For this review, take the finished solid that the model builds, in its own axes (mm). A direction names the side the tool comes from. Give positions to 0.01 mm unless a question says otherwise; leave off trailing zeros. Loops run counter-clockwise (first coordinate to the right, second up) from the corner with the lowest first, then second, coordinate; pieces in that order, holes last.
```python
from build123d import *

# Parameters (mm, degrees)
F0_R     = 3.5
F0_R_2   = 1.5
F1_DEPTH = 2
F0_W     = 22.5
F0_H     = 32
F2_DEPTH = 4
F3_DEPTH = 1


with BuildPart() as f1:
    # F0 (on Top) → F1 (new body)
    with BuildSketch(Plane.XY):
        with BuildLine():
            ThreePointArc((20, 26.114874), (18.904278, 28.704066), (16.409269, 30))
            Line((16.409269, 30), (-16.409269, 30))
            ThreePointArc((-16.409269, 30), (-18.904278, 28.704066), (-20, 26.114874))
            Line((-20, 26.114874), (-20, 24.938533))
            ThreePointArc((-20, 24.938533), (-19.396294, 22.556811), (-17.73096, 20.750233))
            Line((-17.73096, 20.750233), (-13, 17.665434))
            Line((-13, 17.665434), (-13, 18))
            Line((-13, 18), (13, 18))
            Line((13, 18), (13, 17.665434))
            Line((13, 17.665434), (17.73096, 20.750233))
            ThreePointArc((17.73096, 20.750233), (19.396294, 22.556811), (20, 24.938533))
            Line((20, 24.938533), (20, 26.114874))
        make_face()
        with Locations((-15, 25)):
            Circle(F0_R, mode=Mode.SUBTRACT)
        Polygon((-9.18, 27), (-9.18, 28), (-8.18, 28), (8.18, 28), (9.170838, 28), (9.170838, 27), (9.170838, 21), (9.170838, 20), (8.18, 20), (-8.18, 20), (-9.18, 20), (-9.18, 21), align=None, mode=Mode.SUBTRACT)
        with Locations((15, 25)):
            Circle(F0_R, mode=Mode.SUBTRACT)
        with BuildLine():
            Line((17.73096, -20.750233), (13, -17.665434))
            Line((13, -17.665434), (13, -18))
            Line((13, -18), (-13, -18))
            Line((-13, -18), (-13, -17.665434))
            Line((-13, -17.665434), (-17.73096, -20.750233))
            ThreePointArc((-17.73096, -20.750233), (-19.396294, -22.556811), (-20, -24.938533))
            Line((-20, -24.938533), (-20, -26.114874))
            ThreePointArc((-20, -26.114874), (-18.904278, -28.704066), (-16.409269, -30))
            Line((-16.409269, -30), (16.409269, -30))
            ThreePointArc((16.409269, -30), (18.904278, -28.704066), (20, -26.114874))
            Line((20, -26.114874), (20, -24.938533))
            ThreePointArc((20, -24.938533), (19.396294, -22.556811), (17.73096, -20.750233))
        make_face()
        with Locations((-15, -25)):
            Circle(F0_R, mode=Mode.SUBTRACT)
        Polygon((-8.18, -20), (8.18, -20), (9.170838, -20), (9.170838, -21), (9.170838, -27), (9.170838, -28), (8.18, -28), (-8.18, -28), (-9.18, -28), (-9.18, -27), (-9.18, -21), (-9.18, -20), align=None, mode=Mode.SUBTRACT)
        with Locations((15, -25)):
            Circle(F0_R, mode=Mode.SUBTRACT)
        with Locations((-15, -25)):
            Circle(F0_R)
        with Locations((-15, -25)):
            Circle(F0_R_2, mode=Mode.SUBTRACT)
        with Locations((15, -25)):
            Circle(F0_R)
        with Locations((15, -25)):
            Circle(F0_R_2, mode=Mode.SUBTRACT)
        with Locations((15, 25)):
            Circle(F0_R)
        with Locations((15, 25)):
            Circle(F0_R_2, mode=Mode.SUBTRACT)
        with Locations((-15, 25)):
            Circle(F0_R)
        with Locations((-15, 25)):
            Circle(F0_R_2, mode=Mode.SUBTRACT)
        Polygon((-8.18, 28), (-9.18, 28), (-9.18, 27), (-1.743927, 24), (-9.18, 21), (-9.18, 20), (-8.18, 20), (0, 23.300129), (8.18, 20), (9.170838, 20), (9.170838, 21), (1.734764, 24), (9.170838, 27), (9.170838, 28), (8.18, 28), (0, 24.699871), align=None)
        Polygon((9.170838, -20), (8.18, -20), (0, -23.300129), (-8.18, -20), (-9.18, -20), (-9.18, -21), (-1.743927, -24), (-9.18, -27), (-9.18, -28), (-8.18, -28), (0, -24.699871), (8.18, -28), (9.170838, -28), (9.170838, -27), (1.734764, -24), (9.170838, -21), align=None)
    extrude(amount=F1_DEPTH)

    # F0 (on Top) → F2 (join)
    with BuildSketch(Plane.XY):
        Polygon((13, -17.665434), (13, 17.665434), (13, 18), (-13, 18), (-13, 17.665434), (-13, -17.665434), (-13, -18), (13, -18), align=None)
        Rectangle(F0_W, F0_H, mode=Mode.SUBTRACT)
    extrude(amount=F2_DEPTH)

    # F0 (on Top) → F3 (join)
    with BuildSketch(Plane.XY):
        Rectangle(F0_W, F0_H)
    extrude(amount=F3_DEPTH)


solid = f1.part
```
Item 1: Tool access review of faces 4 (the cylindrical face through (-19.38, -22.53, 0.99)), 5 (the flat face through (0, 0, 1)), 6 (the flat face through (15.4, -19.23, 0.99)), 7 (the flat face through (0, -18, 3)), 8 (the flat face through (-5.41, -25.48, 0.99)): name each direction out of +Z, -Z, +X, -X, +Y, -Y from which nothing blocks a thin tool from reaching the whole face with its end or side.
Answer:
face 4: +Z, -Z, -X
face 5: +Z
face 6: +Z, -Z, +X
face 7: +Z, +X, -X, -Y
face 8: +Z, -Z
Item 2: Take a section at C-C on y = -11.5. Give the boundary of the cut face in (x, z), and give its area (3 significant figures).
Answer:
outline: (-13, 0) - (13, 0) - (13, 4) - (11.25, 4) - (11.25, 1) - (-11.25, 1) - (-11.25, 4) - (-13, 4) - close
area: 36.5 mm2
Item 3: Clearance check with flat-ended pins moving along their axes: pin 1 Ø6 at (x, y) = (-8, 23.5) entering from +Z; pin 2 Ø10 at (x, y) = (9.5, 21) entering from +Z; pin 3 Ø2.5 at (x, y) = (15, 25) entering from -Z; pin 4 Ø0.6 at (y, z) = (-22.5, 1) entering from +X. State where each tip first meets the part, or that it passes through.
Answer:
pin 1: stops at z = 2
pin 2: stops at z = 4
pin 3: passes through
pin 4: stops at x = 19.52
Item 4: The part is to be moulded in two halves that separate along Y. For faces 1 (the cylindrical face through (19.38, 22.53, 0.99)), 2 (the flat face through (0, -30, 1)), 3 (the flat face through (0, 30, 1)), say which applies: released by +Y, released by -Y, zero draft, split by the parting line, or undercut.
Answer:
face 1: undercut
face 2: released by -Y
face 3: released by +Y
Item 5: For L1, parallel to Y at x = 15, z = 1.55; L2, parallel to X at y = 11, z = 3.25; L3, parallel to X at y = 26, z = 1.25, list the stretches that pass through material, from the lowest coordinate up.
Answer:
L1: y = -30 to -26.5, -23.5 to -18.97, 18.97 to 23.5, 26.5 to 30
L2: x = -13 to -11.25, 11.25 to 13
L3: x = -20 to -16.12, -13.88 to -9.18, -6.7 to -3.22, 3.22 to 6.69, 9.17 to 13.88, 16.12 to 20
Item 6: Take a section at B-B on x = 15. Give the boundary of the cut face in (y, z).
Answer:
outline: (-30, 0) - (-26.5, 0) - (-26.5, 2) - (-30, 2) - close; (-23.5, 0) - (-18.97, 0) - (-18.97, 2) - (-23.5, 2) - close; (18.97, 0) - (23.5, 0) - (23.5, 2) - (18.97, 2) - close; (26.5, 0) - (30, 0) - (30, 2) - (26.5, 2) - close
Item 7: Take a section at A-A on z = 3.4. Give the boundary of the cut face in (x, y), and give its area (3 significant figures).
Answer:
outline: (-13, -18) - (13, -18) - (13, 18) - (-13, 18) - close; hole (-11.25, -16) - (11.25, -16) - (11.25, 16) - (-11.25, 16) - close
area: 216 mm2
